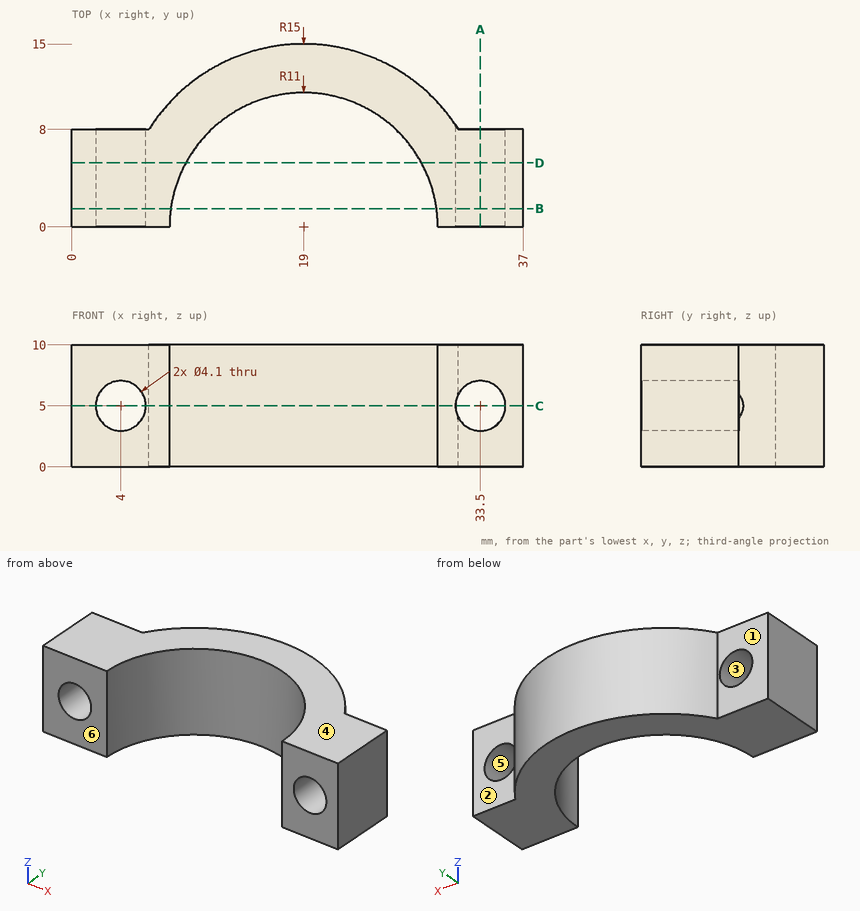
Design review of the part shown in the three views and the two pictorial views. Dimensions are in mm from the part's minimum x, y and z. A direction names the side the tool comes from. Round coordinates to 2 decimals unless told otherwise and drop trailing zeros. Loops run counter-clockwise (first coordinate to the right, second up) from the corner with the lowest first, then second, coordinate; pieces in that order, holes last. Notation, with made-up numbers: (56.5, 83.25) - (102.5, 83.25) arc R11 cw to (102.5, 89.25) - close; hole circle Ø3 at (69, -27.5). An arc over 180 degrees is marked (long way). Write each question's results on one line, items separated by ' | '. Start each with the question number.
Q1. Draft analysis for pull direction Z (two halves, no side actions). For the marked faces 4, 5 and 6, state which applies: pulls with the +Z half, pulls with the -Z half, needs draft (parallel to the pull), parting line crosses it, or undercut.
Q2. Tool access review of the marked faces 1, 2 and 3: name each direction out of +Z, -Z, +X, -X, +Y, -Y from which nothing blocks a thin tool from reaching the whole face with its end or side.
Q3. Take a section at A-A on x = 33.5. Give the boundary of the cut face in (y, z), plus the area to 3 significant figures.
Q4. Take a section at D-D on y = 5.25. Give the boundary of the cut face in (x, z), plus the area to 3 significant figures.
Q5. Insertion check: P1, Ø3, axis at x = 2, z = 5, coming from the +Y side; P2, Ø4, axis at x = 33.5, z = 4, coming from the +Y side; P3, Ø5, axis at x = 13, z = 3, coming from the -Y side. Each pin has a flat end and moves straight along its axis. Give the tip position at first contact, or say it passes through.
Q6. Take a section at C-C on z = 5. Give the boundary of the cut face in (x, y), plus the area to 3 significant figures.
Q7. Take a section at B-B on y = 1.5. Give the boundary of the cut face in (x, z).
Q8. Wall thickness on line 1 along Z through (x, y) = (33.5, 4.75); line 2 along X through (y, z) = (6, 5.5); line 3 along X through (y, z) = (8.25, 6.5): over which ranges is each line inside the solid? List them lowest first. Write a range as [from, to].
Data:
1) face 4: pulls with the +Z half | face 5: undercut | face 6: needs draft
2) face 1: +Z, -Z, -X, +Y | face 2: +Z, -Z, +X, +Y | face 3: +Y, -Y
3) outline: (0, 0) - (8, 0) - (8, 2.95) - (0, 2.95) - close; (0, 7.05) - (8, 7.05) - (8, 10) - (0, 10) - close | area: 47.2 mm²
4) outline: (0, 0) - (9.33, 0) - (9.33, 10) - (0, 10) - close; (28.67, 0) - (37, 0) - (37, 10) - (28.67, 10) - close; hole circle Ø4.1 at (4, 5); hole circle Ø4.1 at (33.5, 5) | area: 150 mm²
5) P1: stops at y = 8 | P2: stops at y = 8.29 | P3: stops at y = 6.98
6) outline: (0, 0) - (1.95, 0) - (1.95, 8) - (0, 8) - close; (6.05, 0) - (8, 0) arc R11 cw to (30, 0) - (31.45, 0) - (31.45, 8.37) arc R15 ccw to (6.31, 8) - (6.05, 8) - close; (35.55, 0) - (37, 0) - (37, 8) - (35.55, 8) - close | area: 166 mm²
7) outline: (0, 0) - (8.1, 0) - (8.1, 10) - (0, 10) - close; (29.9, 0) - (37, 0) - (37, 10) - (29.9, 10) - close; hole circle Ø4.1 at (4, 5); hole circle Ø4.1 at (33.5, 5)
8) line 1: z = [0, 2.95], [7.05, 10] | line 2: x = [0, 2.01], [5.99, 9.78], [28.22, 31.51], [35.49, 37] | line 3: x = [6.47, 11.72], [26.28, 31.53]
